```python
from build123d import *

# Parameters (mm, degrees)
TUBE_SQUARE_40_X_40_X_3_2_4_DEPTH = 1920
SKETCH13_R                        = 2
CUT_EXTRUDE1_DEPTH                = 3


with BuildPart() as part:
    # Sketch12 → Tube (square) 40 X 40 X 3.2(4) (new body)
    with BuildSketch(Plane(origin=(0, 0, 0), x_dir=(0, 0, -1), z_dir=(1, 0, 0))):
        with BuildLine():
            Line((-13.6, -20), (13.6, -20))
            ThreePointArc((13.6, -20), (18.1254834, -18.1254834), (20, -13.6))
            Line((20, -13.6), (20, 13.6))
            ThreePointArc((20, 13.6), (18.1254834, 18.1254834), (13.6, 20))
            Line((13.6, 20), (-13.6, 20))
            ThreePointArc((-13.6, 20), (-18.1254834, 18.1254834), (-20, 13.6))
            Line((-20, 13.6), (-20, -13.6))
            ThreePointArc((-20, -13.6), (-18.1254834, -18.1254834), (-13.6, -20))
        make_face()
        with BuildLine():
            Line((-13.6, -16.8), (13.6, -16.8))
            ThreePointArc((13.6, -16.8), (15.8627417, -15.8627417), (16.8, -13.6))
            Line((16.8, -13.6), (16.8, 13.6))
            ThreePointArc((16.8, 13.6), (15.8627417, 15.8627417), (13.6, 16.8))
            Line((13.6, 16.8), (-13.6, 16.8))
            ThreePointArc((-13.6, 16.8), (-15.8627417, 15.8627417), (-16.8, 13.6))
            Line((-16.8, 13.6), (-16.8, -13.6))
            ThreePointArc((-16.8, -13.6), (-15.8627417, -15.8627417), (-13.6, -16.8))
        make_face(mode=Mode.SUBTRACT)
    extrude(amount=TUBE_SQUARE_40_X_40_X_3_2_4_DEPTH)

    # Sketch13 → Cut-Extrude1 (cut)
    with BuildSketch(Plane(origin=(0, 20, 0), x_dir=(1, 0, 0), z_dir=(0, 1, 0))):
        with Locations(Location((20, 0, 0), (0, 0, 270))):
            Circle(SKETCH13_R)
        with Locations(Location((1900, 0, 0), (0, 0, 270))):
            Circle(SKETCH13_R)
        with Locations(Location((980, 0, 0), (0, 0, 270))):
            Circle(SKETCH13_R)
        with Locations(Location((940, 0, 0), (0, 0, 270))):
            Circle(SKETCH13_R)
        with Locations(Location((1440, 0, 0), (0, 0, 270))):
            Circle(SKETCH13_R)
        with Locations(Location((480, 0, 0), (0, 0, 270))):
            Circle(SKETCH13_R)
    extrude(amount=-CUT_EXTRUDE1_DEPTH, mode=Mode.SUBTRACT)


solid = part.part
```
CAD build for the part. Positions are in the model's coordinates, mm. Round coordinates to 2 decimals unless told otherwise and drop trailing zeros. Loops run counter-clockwise (first coordinate to the right, second up) from the corner with the lowest first, then second, coordinate; pieces in that order, holes last. Notation, with made-up numbers: M -1.75,-6.75 L 23.25,-6.75 A31 ccw 23.25,25.25 Z; hole C 74.5,85 d2. An arc over 180 degrees is marked long. Return JSON: item names as keys, results as strings. Group by question number.
(1) Saw through at A-A, the plane y = 3. List the corners of the cut face in (x, z), and give its area (3 significant figures).
(2) Wall check: probe 1 along Z at (x, y) = (483, 15) (1 decimal); probe 2 along Y at (x, z) = (1258, 2.5); probe 3 along Z at (x, y) = (819, 14.5). Give the ranges that are in metal, low to high. Write a range as [from, to].
(3) Drop flat-ended pins along their axis: P1, Ø4.5, axis at x = 979, z = 0.5, coming from the +Y side; P2, Ø3.5, axis at x = 20, z = 0, coming from the +Y side. Give the stop position or say it passes through.
(4) Saw through at B-B, the plane x = 396. List the corners of the cut face in (y, z), and give its area (3 significant figures).
Answer list:
{
 "1": {"outline": "M 0,-20 L 1920,-20 L 1920,-16.8 L 0,-16.8 Z; M 0,16.8 L 1920,16.8 L 1920,20 L 0,20 Z", "area": "12,300 mm2"},
 "2": {"probe 1": "[-19.8, -16.5], [16.5, 19.8]", "probe 2": "[-20, -16.8], [16.8, 20]", "probe 3": "[-19.94, -16.67], [16.67, 19.94]"},
 "3": {"P1": "y = 20", "P2": "y = 17"},
 "4": {"outline": "M -20,-13.6 A6.4 ccw -13.6,-20 L 13.6,-20 A6.4 ccw 20,-13.6 L 20,13.6 A6.4 ccw 13.6,20 L -13.6,20 A6.4 ccw -20,13.6 Z; hole M -16.8,-13.6 A3.2 ccw -13.6,-16.8 L 13.6,-16.8 A3.2 ccw 16.8,-13.6 L 16.8,13.6 A3.2 ccw 13.6,16.8 L -13.6,16.8 A3.2 ccw -16.8,13.6 Z", "area": "445 mm2"}
}
